from build123d import *

# Parameters (mm, degrees)
SKETCH1_W                              = 100
SKETCH1_H                              = 100
BOSS_EXTRUDE1_DEPTH                    = 20
SKETCH2_R                              = 30
BOSS_EXTRUDE2_DEPTH                    = 70
FILLET1_R                              = 5
CHAMFER1_SIZE                          = 1
FILLET2_R                              = 10
CBORE_FOR_M6_HEX_HEAD_BOLT4_AT_2_COUNT = 2
CBORE_FOR_M6_HEX_HEAD_BOLT4_AT_2_PITCH = 80
CBORE_FOR_M6_HEX_HEAD_BOLT4_AT_3_COUNT = 2
CBORE_FOR_M6_HEX_HEAD_BOLT4_AT_3_PITCH = 113.13708499
CBORE_FOR_M6_HEX_HEAD_BOLT4_AT_4_COUNT = 2
CBORE_FOR_M6_HEX_HEAD_BOLT4_AT_4_PITCH = 80
SKETCH4_R                              = 17.5
CUT_EXTRUDE1_DEPTH                     = 40
SKETCH16_R                             = 22.5
CUT_EXTRUDE2_DEPTH                     = 50


with BuildPart() as part:
    # Sketch1 → Boss-Extrude1 (new body)
    with BuildSketch(Plane.XY):
        with Locations((50, 50)):
            Rectangle(SKETCH1_W, SKETCH1_H)
    extrude(amount=BOSS_EXTRUDE1_DEPTH)

    # Sketch2 → Boss-Extrude2 (add)
    with BuildSketch(Plane.XY.offset(20)):
        with Locations((50, 50)):
            Circle(SKETCH2_R)
    extrude(amount=BOSS_EXTRUDE2_DEPTH)

    # Fillet1
    fillet1_edges = [part.edges().sort_by_distance(p)[0] for p in [
        (20, 50, 20),
    ]]
    fillet(fillet1_edges, radius=FILLET1_R)

    # Chamfer1
    chamfer1_edges = [part.edges().sort_by_distance(p)[0] for p in [
        (20, 50, 90),
    ]]
    chamfer(chamfer1_edges, length=CHAMFER1_SIZE)

    # Fillet2
    fillet2_edges = [part.edges().sort_by_distance(p)[0] for p in [
        (0, 100, 10),
        (100, 100, 10),
        (100, 0, 10),
        (0, 0, 10),
    ]]
    fillet(fillet2_edges, radius=FILLET2_R)

    # Sketch15 → CBORE for M6 Hex Head Bolt4 (revolve, cut)
    with BuildSketch(Plane(origin=(10, 90, 20), x_dir=(0, -1, 0), z_dir=(1, 0, 0))):
        Polygon((0, 0), (0, 20), (3.3, 20), (3.3, 7), (5.5, 7), (5.5, 1.8), (7.3, 0), align=None)
    cbore_for_m6_hex_head_bolt4 = revolve(axis=Axis((10, 90, 26.35), (0, 0, -1)), mode=Mode.SUBTRACT)

    # CBORE for M6 Hex Head Bolt4 at 2: CBORE for M6 Hex Head Bolt4 ×2
    with Locations(*[(0, -i * CBORE_FOR_M6_HEX_HEAD_BOLT4_AT_2_PITCH, 0) for i in range(1, CBORE_FOR_M6_HEX_HEAD_BOLT4_AT_2_COUNT)]):
        add(cbore_for_m6_hex_head_bolt4, mode=Mode.SUBTRACT)

    # CBORE for M6 Hex Head Bolt4 at 3: CBORE for M6 Hex Head Bolt4 ×2
    with Locations(*[Vector(0.7071067811865476, -0.7071067811865475, 0) * (i * CBORE_FOR_M6_HEX_HEAD_BOLT4_AT_3_PITCH) for i in range(1, CBORE_FOR_M6_HEX_HEAD_BOLT4_AT_3_COUNT)]):
        add(cbore_for_m6_hex_head_bolt4, mode=Mode.SUBTRACT)

    # CBORE for M6 Hex Head Bolt4 at 4: CBORE for M6 Hex Head Bolt4 ×2
    with Locations(*[(i * CBORE_FOR_M6_HEX_HEAD_BOLT4_AT_4_PITCH, 0, 0) for i in range(1, CBORE_FOR_M6_HEX_HEAD_BOLT4_AT_4_COUNT)]):
        add(cbore_for_m6_hex_head_bolt4, mode=Mode.SUBTRACT)

    # Sketch4 → Cut-Extrude1 (cut)
    with BuildSketch(Plane.XY.offset(90)):
        with Locations((50, 50)):
            Circle(SKETCH4_R)
    extrude(amount=-CUT_EXTRUDE1_DEPTH, mode=Mode.SUBTRACT)

    # Sketch16 → Cut-Extrude2 (cut)
    with BuildSketch(Plane.XY.offset(50)):
        with Locations((50, 50)):
            Circle(SKETCH16_R)
    extrude(amount=-CUT_EXTRUDE2_DEPTH, mode=Mode.SUBTRACT)


solid = part.part
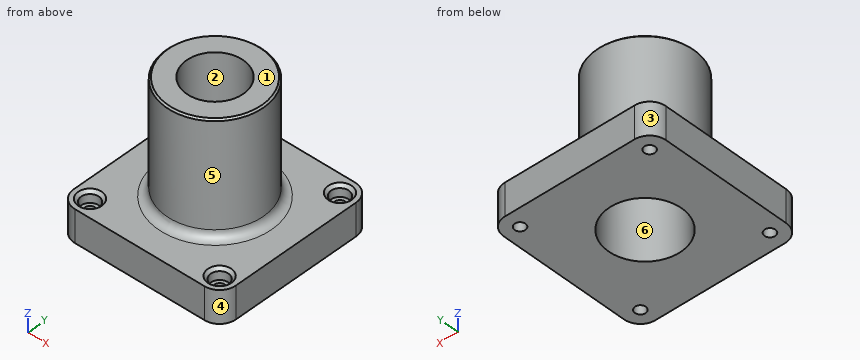
Here's how the part is built. I have some questions about the finished solid (model axes, mm). Face numbers are marked on the shaded views. A direction names the side the tool comes from. Give positions to 0.01 mm unless a question says otherwise; leave off trailing zeros. Order: outer loops, then holes, each group sorted by start corner. A loop starts at its lowest first (then second) coordinate and runs counter-clockwise, first axis right, second up. Notation, with made-up numbers: M -28.5,88.5 L -11.5,88.5 A21 ccw -11.5,126.5 Z; hole C 87.5,89 d5. An arc over 180 degrees is marked long. Answer as a JSON object with one key per item and string values. Group by question number.
1) I'm going to push flat-ended pins straight in: pin 1 Ø5.5 at (x, y) = (90, 10) entering from -Z; pin 2 Ø12 at (x, z) = (37.5, 55.5) entering from +Y; pin 3 Ø5.5 at (x, y) = (8, 9.5) entering from +Z; pin 4 Ø5 at (x, z) = (24, 39) entering from +Y. Where does each tip first touch, or does it pass through?
2) Suppose I cut it at A-A, the plane x = 50. Write out the boundary of the cut face in (y, z).
3) We'd pull the mould along X, two halves only. Please class the marked faces 1, 2 and 3: pulls with the +X half, pulls with the -X half, needs draft (parallel to the pull), parting line crosses it, or undercut.
4) Please list where these lines run through material, in increasing order: L1, parallel to Y at x = 10, z = 16.4; L2, parallel to X at y = 91, z = 10. Write a range as [from, to].
5) Suppose I cut it at C-C, the plane z = 69.5. Write out the boundary of the cut face in (x, y), plus the area to 3 significant figures.
6) Suppose I cut it at D-D, the plane x = 91.5. Count the separate pieces of the cut face and the enclosed holes in it, plus the area to 3 significant figures.
7) On a 3-axis mill with a long thin cutter (end or side, diameter ignored), from which of +Z, -Z, +X, -X, +Y, -Y can I reach the whole of each face in a straight line? I mean the marked faces 4, 5 and 6. Say none if no direction works.
Results found:
{
 "1": {"pin 1": "through", "pin 2": "y = 79.29", "pin 3": "z = 13", "pin 4": "y = 68.65"},
 "2": {"outline": "M 0,0 L 27.5,0 L 27.5,50 L 32.5,50 L 32.5,90 L 21,90 L 20,89 L 20,25 A5 cw 15,20 L 0,20 Z; M 67.5,50 L 72.5,50 L 72.5,0 L 100,0 L 100,20 L 85,20 A5 cw 80,25 L 80,89 L 79,90 L 67.5,90 Z"},
 "3": {"face 1": "needs draft", "face 2": "undercut", "face 3": "pulls with the -X half"},
 "4": {"L1": "[0, 4.5], [15.5, 84.5], [95.5, 100]", "L2": "[0.05, 6.86], [13.14, 86.86], [93.14, 99.95]"},
 "5": {"outline": "C 50,50 d60; hole C 50,50 d35", "area": "1,870 mm²"},
 "6": {"separate pieces": "3", "enclosed holes": "0", "area": "1,690 mm²"},
 "7": {"face 4": "+Z, -Z, +X, -Y", "face 5": "+Z", "face 6": "-Z"}
}
